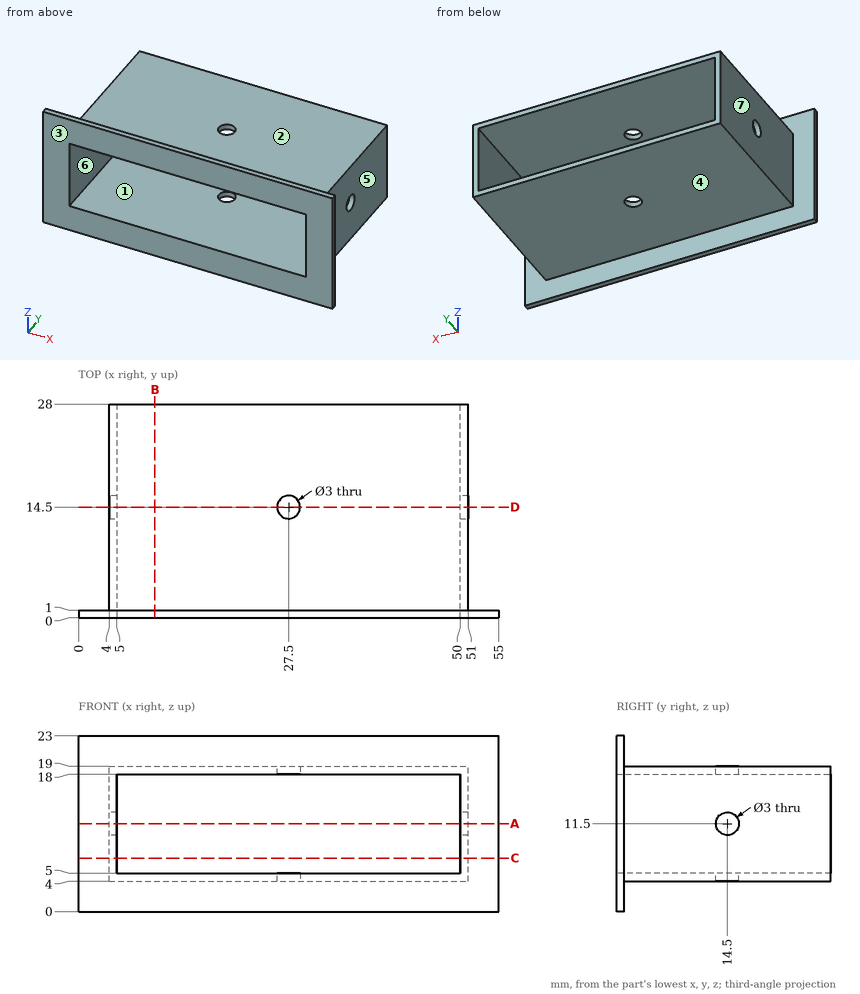
Here's the drawing with two shaded views (mm, measured from the low corner). I have some questions. A direction names the side the tool comes from. Coordinates: 2 decimals unless noted, no trailing zeros. Loops run counter-clockwise (first coordinate to the right, second up) from the corner with the lowest first, then second, coordinate; pieces in that order, holes last. Notation, with made-up numbers: M -38,-20 L -16,-20 A27 ccw -16,9 Z; hole C 37.25,21.5 d6. An arc over 180 degrees is marked long. Put each result on its own line as item: value. Start each with the question number.
(1) I need wall thicknesses on probe 1 along X at (y, z) = (10.75, 14); probe 2 along Z at (x, y) = (15.5, 5); probe 3 along Y at (x, z) = (17, 1.25). Which ranges of each line are inside material? Lowest first, please.
(2) We'd pull the mould along X, two halves only. Please class the marked faces 5, 6 and 7: +X half, -X half, draft (parallel to the pull), parting line (faces both ways), or undercut.
(3) Imagine slicing it at B-B on x = 10. List the corners of the cut face in (y, z) for me, and give its area (3 significant figures).
(4) Imagine slicing it at A-A on z = 11.5. List the corners of the cut face in (x, y) for me.
(5) Imagine slicing it at D-D on y = 14.5. List the corners of the cut face in (x, z) for me, and give its area (3 significant figures).
(6) Will these pins go through, and if not, where does the flat tip stop? pin 1 Ø12 at (x, y) = (29, 23.5) entering from -Z; pin 2 Ø2 at (y, z) = (21.5, 14) entering from +X; pin 3 Ø5 at (x, y) = (19.5, 12) entering from +Z.
(7) Imagine slicing it at C-C on z = 7. List the corners of the cut face in (x, y) for me.
(8) Which directions (+Z, -Z, +X, -X, +Y, -Y) give clear straight access to the entire face, cutting with the end or side of a thin tool? Please do the marked faces 1, 2, 3 and 4.
Worked answers:
1. probe 1: x = 4 to 5, 50 to 51
1. probe 2: z = 4 to 5, 18 to 19
1. probe 3: y = 0 to 1
2. face 5: +X half
2. face 6: undercut
2. face 7: -X half
3. outline: M 0,0 L 1,0 L 1,4 L 28,4 L 28,5 L 0,5 Z; M 0,18 L 28,18 L 28,19 L 1,19 L 1,23 L 0,23 Z
3. area: 64.0 mm2
4. outline: M 0,0 L 5,0 L 5,13 L 4,13 L 4,1 L 0,1 Z; M 4,16 L 5,16 L 5,28 L 4,28 Z; M 50,0 L 55,0 L 55,1 L 51,1 L 51,13 L 50,13 Z; M 50,16 L 51,16 L 51,28 L 50,28 Z
5. outline: M 4,4 L 26,4 L 26,5 L 5,5 L 5,10 L 4,10 Z; M 4,13 L 5,13 L 5,18 L 26,18 L 26,19 L 4,19 Z; M 29,4 L 51,4 L 51,10 L 50,10 L 50,5 L 29,5 Z; M 29,18 L 50,18 L 50,13 L 51,13 L 51,19 L 29,19 Z
5. area: 108 mm2
6. pin 1: stops at z = 4
6. pin 2: stops at x = 51
6. pin 3: stops at z = 19
7. outline: M 0,0 L 5,0 L 5,28 L 4,28 L 4,1 L 0,1 Z; M 50,0 L 55,0 L 55,1 L 51,1 L 51,28 L 50,28 Z
8. face 1: +Y, -Y
8. face 2: +Z, +X, -X, +Y
8. face 3: +Z, -Z, +X, -X, -Y
8. face 4: -Z, +X, -X, +Y
